Input: part model. Units: mm. Frame: model coordinates. Round coordinates to 2 decimals unless told otherwise and drop trailing zeros.
Item 1: Line query: L1, parallel to X at y = 438.15, z = 1.75; L2, parallel to Y at x = 1168.4, z = 2.5; L3, parallel to X at y = 18, z = 2.75. Output: solid intervals per line, ascending.
Item 2: First-contact query: pin 1 (3 mm diameter, centred on y = 12.5, z = 4.5, fed in from -X); pin 2 (1.9 mm diameter, centred on x = 496.5, z = 2.5, fed in from -Y); pin 3 (3 mm diameter, centred on x = 49.5, z = 2, fed in from -Y). Flat tips, straight axial feed; report the tip coordinate or a pass-through.
Item 3: Cut plane A-A on z = 5. Give the number of separate pieces and of enclosed holes in the cut face, then the cut area to 3 significant figures.
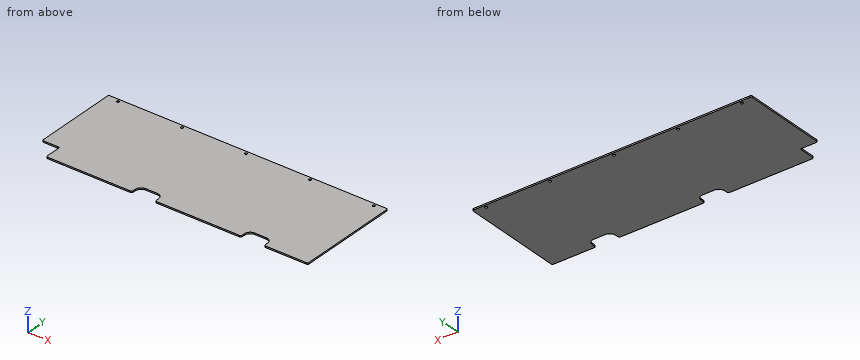
```python
from build123d import *

# Parameters (mm, degrees)
SKETCH1_W                        = 1219.2
SKETCH1_H                        = 450.85
BOSS_EXTRUDE1_DEPTH              = 6.35
CUT_EXTRUDE1_DEPTH               = 1300.905644653
LPATTERN1_COUNT                  = 2
LPATTERN1_PITCH                  = 476.25
SKETCH3_W                        = 76.2
SKETCH3_H                        = 76.2
CUT_EXTRUDE2_DEPTH               = 1300.905644653
FILLET1_R                        = 6.35
F_27_64_0_42188_DIAMETER_HOLE1_D = 10.715752
FILLET2_R                        = 6.35


with BuildPart() as part:
    # Sketch1 → Boss-Extrude1 (new body)
    with BuildSketch(Plane.XY):
        with Locations((609.6, 225.425)):
            Rectangle(SKETCH1_W, SKETCH1_H)
    extrude(amount=BOSS_EXTRUDE1_DEPTH)

    # Sketch2 → Cut-Extrude1 (cut, through all)
    with BuildSketch(Plane.XY.offset(6.35)):
        with BuildLine():
            Line((450.85, 19.05), (450.85, 0))
            Line((450.85, 0), (552.45, 0))
            Line((552.45, 0), (552.45, 19.05))
            ThreePointArc((552.45, 19.05), (545.010512242, 37.010512242), (527.05, 44.45))
            Line((527.05, 44.45), (476.25, 44.45))
            ThreePointArc((476.25, 44.45), (458.289487758, 37.010512242), (450.85, 19.05))
        make_face()
    cut_extrude1 = extrude(amount=-CUT_EXTRUDE1_DEPTH, mode=Mode.SUBTRACT)

    # LPattern1: Cut-Extrude1 ×2
    with Locations(*[(i * LPATTERN1_PITCH, 0, 0) for i in range(1, LPATTERN1_COUNT)]):
        add(cut_extrude1, mode=Mode.SUBTRACT)

    # Sketch3 → Cut-Extrude2 (cut, through all)
    with BuildSketch(Plane.XY.offset(6.35)):
        with Locations((38.1, 38.1)):
            Rectangle(SKETCH3_W, SKETCH3_H)
    extrude(amount=-CUT_EXTRUDE2_DEPTH, mode=Mode.SUBTRACT)

    # Fillet1
    fillet1_edges = [part.edges().sort_by_distance(p)[0] for p in [
        (76.2, 76.2, 3.175),
    ]]
    fillet(fillet1_edges, radius=FILLET1_R)

    # 27/64 (0.42188) Diameter Hole1 (through all)
    with Locations(Plane.XY.offset(6.35)):
        with Locations((50.8, 438.15), (330.2, 438.15), (609.6, 438.15), (889, 438.15), (1168.4, 438.15)):
            Hole(F_27_64_0_42188_DIAMETER_HOLE1_D / 2)

    # Fillet2
    fillet2_edges = [part.edges().sort_by_distance(p)[0] for p in [
        (552.45, 0, 3.175),
        (450.85, 0, 3.175),
        (1028.7, 0, 3.175),
        (927.1, 0, 3.175),
        (0, 76.2, 3.175),
        (76.2, 0, 3.175),
        (0, 450.85, 3.175),
        (1219.2, 450.85, 3.175),
        (1219.2, 0, 3.175),
    ]]
    fillet(fillet2_edges, radius=FILLET2_R)


solid = part.part
```
From the geometry:
1. L1: x = 0 to 45.44, 56.16 to 324.84, 335.56 to 604.24, 614.96 to 883.64, 894.36 to 1163.04, 1173.76 to 1219.2
1. L2: y = 0 to 432.79, 443.51 to 450.85
1. L3: x = 76.2 to 450.85, 552.45 to 927.1, 1028.7 to 1219.2
2. pin 1: stops at x = 76.2
2. pin 2: stops at y = 44.45
2. pin 3: stops at y = 76.2
3. separate pieces: 1
3. enclosed holes: 5
3. area: 535,000 mm2
